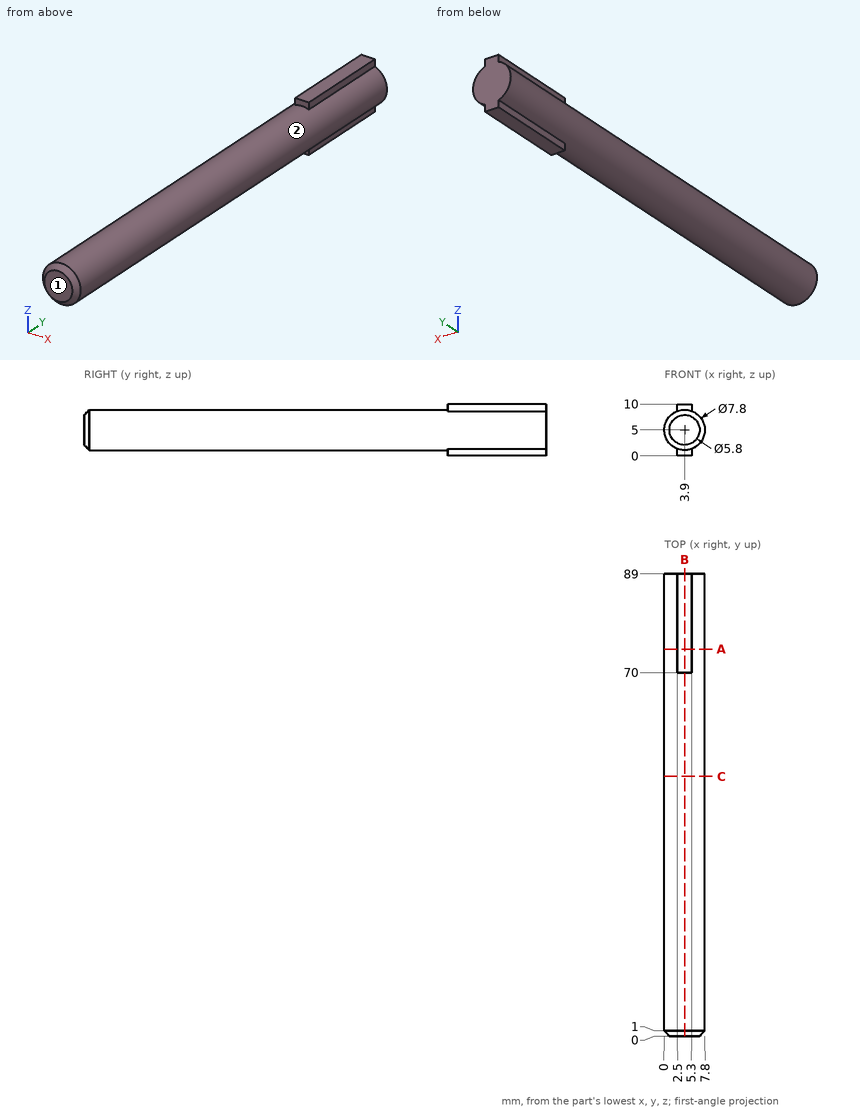
For this review, use the dimensioned drawing (mm, ordinates from the lowest corner) and the shaded views. A direction names the side the tool comes from. Give positions to 0.01 mm unless a question says otherwise; leave off trailing zeros. Order: outer loops, then holes, each group sorted by start corner. A loop starts at its lowest first (then second) coordinate and runs counter-clockwise, first axis right, second up. Notation, with made-up numbers: (-34.5, 69.5) - (20.5, 69.5) arc R35 ccw to (20.5, 104.5) - close; hole circle Ø3 at (76, 9.5). An arc over 180 degrees is marked (long way). Use a Markdown table: item, result. Add a question column.
(1) Wall thickness on probe 1 along Z at (x, y) = (6.5, 51); probe 2 along Z at (x, y) = (5.25, 14); probe 3 along Y at (x, z) = (3, 1): over which ranges is each line inside the solid? List them lowest first. Write a range as [from, to].
(2) Add section B-B on x = 3.9. Give the boundary of the cut face in (y, z), then the cut area to 3 significant figures.
(3) Machinability: for the marked faces 1 and 2, which of the approach directions +Z, -Z, +X, -X, +Y, -Y give a long, thin tool a straight path to every point of the face, cutting with its end or side? Answer none if there is none.
(4) Add section A-A on y = 74.5. Give the boundary of the cut face in (x, z), then the cut area to 3 significant figures.
(5) Add section C-C on y = 50. Give the boundary of the cut face in (x, z), then the cut area to 3 significant figures.
(6) Clearance check with flat-ended pins moving along their axes: P1, Ø1.5, axis at y = 32.5, z = 7, coming from the +X side; P2, Ø3, axis at x = 5.5, y = 64, coming from the -Z side; P3, Ø4, axis at x = 2.5, y = 45, coming from the +Z side. State where each tip first meets the part, or that it passes through.
Report:
| question | item | result |
|---|---|---|
| 1 | probe 1 | z = [2.09, 7.91] |
| 1 | probe 2 | z = [1.34, 8.66] |
| 1 | probe 3 | y = [70, 89] |
| 2 | outline | (0, 2.1) - (1, 1.1) - (70, 1.1) - (70, 0) - (89, 0) - (89, 10) - (70, 10) - (70, 8.9) - (1, 8.9) - (0, 7.9) - close |
| 2 | area | 735 mm² |
| 3 | face 1 | +Z, -Z, +X, -X, -Y |
| 3 | face 2 | -Y |
| 4 | outline | (2.5, 0) - (5.3, 0) - (5.3, 1.36) arc R3.9 ccw to (5.3, 8.64) - (5.3, 10) - (2.5, 10) - (2.5, 8.64) arc R3.9 ccw to (2.5, 1.36) - close |
| 4 | area | 54.4 mm² |
| 5 | outline | circle Ø7.8 at (3.9, 5) |
| 5 | area | 47.8 mm² |
| 6 | P1 | stops at x = 7.59 |
| 6 | P2 | stops at z = 1.1 |
| 6 | P3 | stops at z = 8.9 |
